Check sheet for the modelled part. Datum: model origin and axes. Units: mm. Round coordinates to 2 decimals unless told otherwise and drop trailing zeros. Write each loop counter-clockwise with the first axis right and the second up, starting at its lowest first coordinate (ties: lowest second). Pieces come first, ordered by that corner, then holes.
Item 1: Go/stop test with flat-tipped pins: pin 1 Ø12 at (x, z) = (-4.5, 9.5) entering from -Y; pin 2 Ø1 at (x, y) = (1.5, -3.5) entering from +Z; pin 3 Ø1.8 at (x, y) = (10, -14) entering from +Z; pin 4 Ø1.6 at (y, z) = (-14, 2.5) entering from +X. Record where each tip stops, or that it passes through.
Item 2: Material ranges on line 1 (Y direction, x = -12, z = 2.5); line 2 (Y direction, x = -5, z = 2.5); line 3 (Z direction, x = -11.5, y = -11.5), recorded low to high.
Item 3: Cross-section at B-B on x = -13. Enter the section's corners in (y, z), plus the area to 3 significant figures.
Item 4: Cross-section at A-A on x = -9.25. Enter the section's corners in (y, z), plus the area to 3 significant figures.
Item 5: Cross-section at C-C on z = 30. Enter the section's corners in (x, y).
Item 6: Cross-section at D-D on y = -5. Enter the section's corners in (x, z), plus the area to 3 significant figures.
from build123d import *

# Parameters (mm, degrees)
SKETCH1_W           = 32.5
SKETCH1_H           = 37
BOSS_EXTRUDE1_DEPTH = 2
SKETCH2_W           = 3
SKETCH2_H           = 1.6
BOSS_EXTRUDE2_DEPTH = 1.5
SKETCH3_W           = 7
SKETCH3_H           = 7
CUT_EXTRUDE1_DEPTH  = 4.5
FILLET1_R           = 2
SKETCH4_W           = 32.5
SKETCH4_H           = 39
BOSS_EXTRUDE3_DEPTH = 2
CUT_EXTRUDE2_DEPTH  = 2


with BuildPart() as part:
    # Sketch1 → Boss-Extrude1 (new body)
    with BuildSketch(Plane.XY):
        Rectangle(SKETCH1_W, SKETCH1_H)
    extrude(amount=BOSS_EXTRUDE1_DEPTH)

    # Sketch2 → Boss-Extrude2 (add)
    with BuildSketch(Plane.XY.offset(2)):
        with Locations((-12.75, -13.65)):
            Rectangle(SKETCH2_W, SKETCH2_H)
        with Locations((9.25, -13.65)):
            Rectangle(SKETCH2_W, SKETCH2_H)
    extrude(amount=BOSS_EXTRUDE2_DEPTH)

    # Sketch3 → Cut-Extrude1 (cut, through all)
    with BuildSketch(Plane(origin=(0, 0, 0), x_dir=(-1, 0, 0), z_dir=(0, 0, -1))):
        with Locations((2.75, -12)):
            Rectangle(SKETCH3_W, SKETCH3_H)
    extrude(amount=-CUT_EXTRUDE1_DEPTH, mode=Mode.SUBTRACT)

    # Fillet1
    fillet1_edges = [part.edges().sort_by_distance(p)[0] for p in [
        (0.75, -15.5, 1),
        (0.75, -8.5, 1),
        (-6.25, -8.5, 1),
        (-6.25, -15.5, 1),
    ]]
    fillet(fillet1_edges, radius=FILLET1_R)

    # Sketch4 → Boss-Extrude3 (add)
    with BuildSketch(Plane(origin=(0, 18.5, 0), x_dir=(1, 0, 0), z_dir=(0, 1, 0))):
        with Locations((0, -19.5)):
            Rectangle(SKETCH4_W, SKETCH4_H)
    extrude(amount=BOSS_EXTRUDE3_DEPTH)

    # Sketch5 → Cut-Extrude2 (cut)
    with BuildSketch(Plane(origin=(0, 20.5, 0), x_dir=(1, 0, 0), z_dir=(0, 1, 0))):
        with BuildLine():
            Line((-10.75, -24), (-10.75, -14))
            ThreePointArc((-10.75, -14), (-9.25, -12.5), (-7.75, -14))
            Line((-7.75, -14), (-7.75, -24))
            ThreePointArc((-7.75, -24), (-9.25, -25.5), (-10.75, -24))
        make_face()
    extrude(amount=-CUT_EXTRUDE2_DEPTH, mode=Mode.SUBTRACT)


solid = part.part
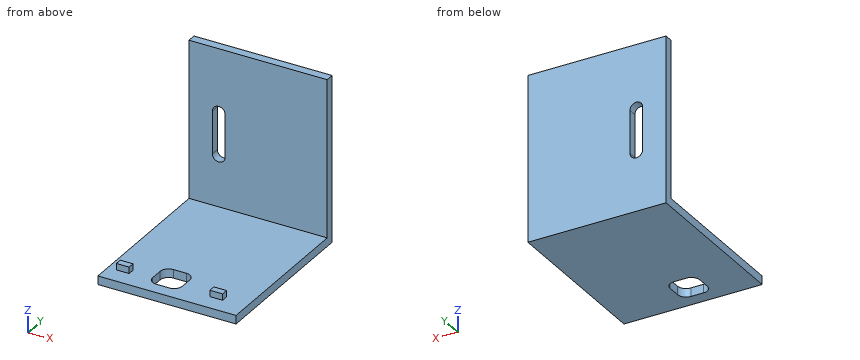
Response values:
1. pin 1: stops at y = 18.5
1. pin 2: stops at z = 2
1. pin 3: stops at z = 3.5
1. pin 4: stops at x = 16.25
2. line 1: y = -14.45 to -12.85, 18.5 to 20.5
2. line 2: y = 18.5 to 20.5
2. line 3: z = 0 to 2
3. outline: (-18.5, 0) - (20.5, 0) - (20.5, 39) - (18.5, 39) - (18.5, 2) - (-12.85, 2) - (-12.85, 3.5) - (-14.45, 3.5) - (-14.45, 2) - (-18.5, 2) - close
3. area: 154 mm2
4. outline: (-18.5, 0) - (20.5, 0) - (20.5, 12.5) - (18.5, 12.5) - (18.5, 2) - (-18.5, 2) - close; (18.5, 25.5) - (20.5, 25.5) - (20.5, 39) - (18.5, 39) - close
4. area: 126 mm2
5. outline: (-16.25, 18.5) - (16.25, 18.5) - (16.25, 20.5) - (-16.25, 20.5) - close
6. outline: (-16.25, 0) - (16.25, 0) - (16.25, 2) - (-16.25, 2) - close
6. area: 65.0 mm2
